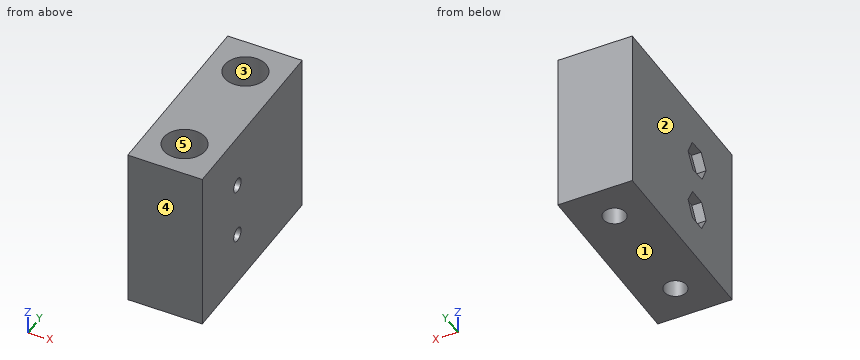
from build123d import *

# Parameters (mm, degrees)
F0_W     = 32.512
F0_H     = 27.94
F1_DEPTH = 12.7
F2_R     = 1.2065
F3_DEPTH = 12.701
F5_DEPTH = 1.651
F6_R     = 1.905
F7_DEPTH = 27.941
F8_R     = 3.556
F9_DEPTH = 18.415


with BuildPart() as f1:
    # F0 (on Right) → F1 (new body)
    with BuildSketch(Plane.YZ):
        with Locations((0, 4.445)):
            Rectangle(F0_W, F0_H)
    extrude(amount=F1_DEPTH)

    # F2 (on face) → F3 (cut, through all)
    with BuildSketch(Plane(origin=(0, 0, 0), x_dir=(0, -1, 0), z_dir=(-1, 0, 0))):
        with Locations((4.826, -0.3048)):
            Circle(F2_R)
        with Locations((4.826, 9.1948)):
            Circle(F2_R)
    extrude(amount=-F3_DEPTH, mode=Mode.SUBTRACT)

    # F4 (on face) → F5 (cut)
    with BuildSketch(Plane(origin=(0, 0, 0), x_dir=(0, -1, 0), z_dir=(-1, 0, 0))):
        Polygon((7.754274, 9.360161), (6.14693, 11.81344), (3.218656, 11.648079), (1.897726, 9.029439), (3.50507, 6.57616), (6.433344, 6.741521), align=None)
        Polygon((6.29247, 2.2352), (3.35953, 2.2352), (1.893061, -0.3048), (3.35953, -2.8448), (6.29247, -2.8448), (7.758939, -0.3048), align=None)
    extrude(amount=-F5_DEPTH, mode=Mode.SUBTRACT)

    # F6 (on face) → F7 (cut, through all)
    with BuildSketch(Plane.XY.offset(18.415)):
        with Locations((6.35, -9.906)):
            Circle(F6_R)
        with Locations((6.35, 9.906)):
            Circle(F6_R)
    extrude(amount=-F7_DEPTH, mode=Mode.SUBTRACT)

    # F8 (on face) → F9 (cut)
    with BuildSketch(Plane.XY.offset(18.415)):
        with Locations((6.35, 9.906)):
            Circle(F8_R)
        with Locations((6.35, -9.906)):
            Circle(F8_R)
    extrude(amount=-F9_DEPTH, mode=Mode.SUBTRACT)


solid = f1.part
Verification items for the finished model (mm, model axes). Face numbers are marked on the shaded views. A direction names the side the tool comes from. Give positions to 0.01 mm unless a question says otherwise; leave off trailing zeros. Loops run counter-clockwise (first coordinate to the right, second up) from the corner with the lowest first, then second, coordinate; pieces in that order, holes last.
1) Sectioned sample at C-C, the plane x = 3.5. Enter the section's corners in (y, z) (1 decimal), then the cut area to 3 significant figures.
2) Set-up check for the marked faces 4 and 5: record each of +Z, -Z, +X, -X, +Y, -Y from which the full face is reachable in a straight line by a thin tool's end or side.
3) Sectioned sample at A-A, the plane x = 6.75. Enter the section's corners in (y, z) (1 decimal).
4) Thickness scan on line 1 along Y through (x, z) = (6.35, 6.25); line 2 along Y through (x, z) = (5, 3.75); line 3 along Y through (x, z) = (9.5, 10.25). Record the ranges inside material, lowest first.
5) Sectioned sample at D-D, the plane z = 5.25. Enter the section's corners in (x, y), then the cut area to 3 significant figures.
6) Draft check along X on the marked faces 1, 2 and 3. Enter one of: pulls with the +X half, pulls with the -X half, needs draft (parallel to the pull), parting line crosses it, or undercut.
7) Sectioned sample at B-B, the plane z = -7.5. Enter the section's corners in (x, y) (3 decimals), then the cut area to 3 significant figures.
8) Depth check by flat-ended pin: pin 1 Ø1.6 at (y, z) = (-4, 10) entering from -X; pin 2 Ø2 at (x, y) = (8, 10.5) entering from +Z. Enter the tip coordinate at first touch or a pass-through.
Answers:
1. outline: (-16.3, -9.5) - (16.3, -9.5) - (16.3, 18.4) - (12, 18.4) - (12, 0) - (7.8, 0) - (7.8, 18.4) - (-7.8, 18.4) - (-7.8, 0) - (-12, 0) - (-12, 18.4) - (-16.3, 18.4) - close; hole circle Ø2.4 at (-4.8, -0.3); hole circle Ø2.4 at (-4.8, 9.2)
1. area: 743 mm2
2. face 4: +Z, -Z, +X, -X, -Y
2. face 5: +Z
3. outline: (-16.3, -9.5) - (-11.8, -9.5) - (-11.8, 0) - (-13.4, 0) - (-13.4, 18.4) - (-16.3, 18.4) - close; (-8, -9.5) - (8, -9.5) - (8, 0) - (6.4, 0) - (6.4, 18.4) - (-6.4, 18.4) - (-6.4, 0) - (-8, 0) - close; (11.8, -9.5) - (16.3, -9.5) - (16.3, 18.4) - (13.4, 18.4) - (13.4, 0) - (11.8, 0) - close; hole circle Ø2.4 at (-4.8, -0.3); hole circle Ø2.4 at (-4.8, 9.2)
4. line 1: y = -16.26 to -13.46, -6.35 to 6.35, 13.46 to 16.26
4. line 2: y = -16.26 to -13.2, -6.62 to 6.62, 13.2 to 16.26
4. line 3: y = -16.26 to -11.56, -8.26 to -5.41, -4.24 to 8.26, 11.56 to 16.26
5. outline: (0, -16.26) - (12.7, -16.26) - (12.7, 16.26) - (0, 16.26) - close; hole circle Ø7.11 at (6.35, -9.91); hole circle Ø7.11 at (6.35, 9.91)
5. area: 333 mm2
6. face 1: needs draft
6. face 2: pulls with the -X half
6. face 3: undercut
7. outline: (0, -16.256) - (12.7, -16.256) - (12.7, 16.256) - (0, 16.256) - close; hole circle Ø3.81 at (6.35, -9.906); hole circle Ø3.81 at (6.35, 9.906)
7. area: 390 mm2
8. pin 1: stops at x = 1.65
8. pin 2: stops at z = 0
